Could you check a few things on this model? Use its own coordinates, in mm. Face numbers are marked on the shaded views. A direction names the side the tool comes from. Round coordinates to 2 decimals unless told otherwise and drop trailing zeros. Write each loop counter-clockwise with the first axis right and the second up, starting at its lowest first coordinate (ties: lowest second). Pieces come first, ordered by that corner, then holes. Notation, with made-up numbers: (9.5, -11.75) -> (52.5, -11.75) arc R26 cw to (52.5, 8.25) -> close; hole circle Ø9 at (14.25, -13). An arc over 180 degrees is marked (long way). Answer in a Markdown table with one row per item.
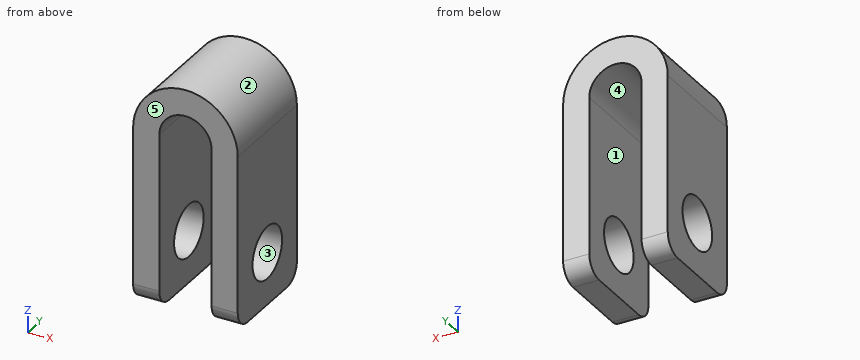
from build123d import *

# Parameters (mm, degrees)
F1_DEPTH = 6
F3_D     = 3
F4_R     = 1


# Not quite as in the source:
# - a feature names something its author has since deleted; it is built from what else it names


with BuildPart() as f1:
    # F0 (on Front) → F1 (new body)
    with BuildSketch(Plane.XZ):
        with BuildLine():
            Line((-1.5, -10), (-1.5, 0))
            ThreePointArc((-1.5, 0), (0, 1.5), (1.5, 0))
            Line((1.5, 0), (1.5, -10))
            Line((1.5, -10), (3, -10))
            Line((3, -10), (3, 0))
            ThreePointArc((3, 0), (0, 3), (-3, 0))
            Line((-3, 0), (-3, -10))
            Line((-3, -10), (-1.5, -10))
        make_face()
    extrude(amount=F1_DEPTH)

    # F3 (through all)
    with Locations(Plane(origin=(-3, 0, 0), x_dir=(0, -1, 0), z_dir=(-1, 0, 0))):
        with Locations((3, -7)):
            Hole(F3_D / 2)

    # F4
    f4_edges = [f1.edges().sort_by_distance(p)[0] for p in [
        (-2.25, -6, -10),
        (2.25, -6, -10),
        (2.25, 0, -10),
        (-2.25, 0, -10),
    ]]
    fillet(f4_edges, radius=F4_R)


solid = f1.part
1) Imagine slicing it at D-D, the plane x = 2.2. Please give me the cut outline in (y, z).
Findings:
| item | result |
|---|---|
| outline | (-6, -9) arc R1 ccw to (-5, -10) -> (-1, -10) arc R1 ccw to (0, -9) -> (0, 2.04) -> (-6, 2.04) -> close; hole circle Ø3 at (-3, -7) |
2) For pin 1 (2 mm diameter, centred on x = -1.5, y = -1.5, fed in from +Z); pin 2 (1.5 mm diameter, centred on x = -2.5, z = 1.5, fed in from +Y); pin 3 (2.5 mm diameter, centred on y = -3, z = -7, fed in from -X); pin 4 (1.5 mm diameter, centred on x = 1.5, y = -5, fed in from +Z), each with a flat end and sliding along its axis, tell me the tip position at first contact or that it passes through.
Findings:
| item | result |
|---|---|
| pin 1 | stops at z = 2.96 |
| pin 2 | stops at y = 0 |
| pin 3 | passes through |
| pin 4 | stops at z = 2.9 |
3) For the marked faces 1 and 2, which set-ups out of +Z, -Z, +X, -X, +Y, -Y let a thin tool reach every point of the face, with its end or its side?
Findings:
| item | result |
|---|---|
| face 1 | -Z, +Y, -Y |
| face 2 | +Z, +Y, -Y |
4) Imagine slicing it at B-B, the plane z = -0.25. Please give me the cut outline in (x, y), plus the area to 3 significant figures.
Findings:
| item | result |
|---|---|
| outline | (-3, -6) -> (-1.5, -6) -> (-1.5, 0) -> (-3, 0) -> close; (1.5, -6) -> (3, -6) -> (3, 0) -> (1.5, 0) -> close |
| area | 18.0 mm^2 |
5) Thinking about a two-plate mould opening in Z: for the marked faces 3, 4 and 5, which applies, +Z half, -Z half, draft (parallel to the pull), parting line (faces both ways), or undercut?
Findings:
| item | result |
|---|---|
| face 3 | undercut |
| face 4 | -Z half |
| face 5 | draft |
6) Imagine slicing it at C-C, the plane y = -2.1. Please give me the cut outline in (x, z), plus the area to 3 significant figures.
Findings:
| item | result |
|---|---|
| outline | (-3, -10) -> (-1.5, -10) -> (-1.5, -8.2) -> (-3, -8.2) -> close; (-3, -5.8) -> (-1.5, -5.8) -> (-1.5, 0) arc R1.5 cw to (1.5, 0) -> (1.5, -5.8) -> (3, -5.8) -> (3, 0) arc R3 ccw to (-3, 0) -> close; (1.5, -10) -> (3, -10) -> (3, -8.2) -> (1.5, -8.2) -> close |
| area | 33.4 mm^2 |
7) Imagine slicing it at A-A, the plane y = -3. Please give me the cut outline in (x, z).
Findings:
| item | result |
|---|---|
| outline | (-3, -10) -> (-1.5, -10) -> (-1.5, -8.5) -> (-3, -8.5) -> close; (-3, -5.5) -> (-1.5, -5.5) -> (-1.5, 0) arc R1.5 cw to (1.5, 0) -> (1.5, -5.5) -> (3, -5.5) -> (3, 0) arc R3 ccw to (-3, 0) -> close; (1.5, -10) -> (3, -10) -> (3, -8.5) -> (1.5, -8.5) -> close |
8) Please list where these lines run through material, in increasing order: line 1 (X direction, y = -0.3, z = -3); line 2 (X direction, y = -1.6, z = 1); line 3 (Z direction, x = -2.5, y = -3).
Findings:
| item | result |
|---|---|
| line 1 | x = -3 to -1.5, 1.5 to 3 |
| line 2 | x = -2.83 to -1.12, 1.12 to 2.83 |
| line 3 | z = -10 to -8.5, -5.5 to 1.66 |
